from build123d import *

# Parameters (mm, degrees)
SKETCH2_W           = 121.6
SKETCH2_H           = 98.919653249
SKETCH2_R           = 2
BOSS_EXTRUDE1_DEPTH = 3
SKETCH3_W           = 3
SKETCH3_H           = 12.364956656
BOSS_EXTRUDE2_DEPTH = 3
CUT_EXTRUDE1_DEPTH  = 101.7


with BuildPart() as part:
    # Sketch2 → Boss-Extrude1 (new body)
    with BuildSketch(Plane(origin=(0, 0, 0), x_dir=(1, 0, 0), z_dir=(0, 1, 0))):
        with Locations((20.5, -5.540173376)):
            Rectangle(SKETCH2_W, SKETCH2_H)
        Polygon((41.25, 0), (0, 0), (0, 7.75), (-2, 7.75), (-3, 10.25), (-2, 12.75), (0, 12.75), (0, 20.5), (41.25, 20.5), align=None, mode=Mode.SUBTRACT)
        with Locations(Location((-4.7, 4.7, 0), (0, 0, 270))):
            Circle(SKETCH2_R, mode=Mode.SUBTRACT)
        with Locations(Location((-4.7, 15.8, 0), (0, 0, 270))):
            Circle(SKETCH2_R, mode=Mode.SUBTRACT)
        with Locations(Location((45.7, 4.7, 0), (0, 0, 270))):
            Circle(SKETCH2_R, mode=Mode.SUBTRACT)
        with Locations(Location((45.7, 15.8, 0), (0, 0, 270))):
            Circle(SKETCH2_R, mode=Mode.SUBTRACT)
    extrude(amount=BOSS_EXTRUDE1_DEPTH)

    # Sketch3 → Boss-Extrude2 (add, through all)
    with BuildSketch(Plane(origin=(0, 0, 0), x_dir=(1, 0, 0), z_dir=(0, 1, 0))):
        with Locations((-41.8, 26.736608875)):
            Rectangle(SKETCH3_W, SKETCH3_H)
        with Locations((-41.8, -6.236608875)):
            Rectangle(SKETCH3_W, SKETCH3_H)
        with Locations((82.8, -6.236608875)):
            Rectangle(SKETCH3_W, SKETCH3_H)
        with Locations((82.8, 26.736608875)):
            Rectangle(SKETCH3_W, SKETCH3_H)
    extrude(amount=BOSS_EXTRUDE2_DEPTH)

    # Sketch4 → Cut-Extrude1 (cut, through all)
    with BuildSketch(Plane(origin=(0, 0, 0), x_dir=(1, 0, 0), z_dir=(0, 1, 0))):
        Polygon((81.3, 8.75), (74.3, 8.75), (74.3, 7.25), (72.3, 7.25), (72.3, 13.25), (74.3, 13.25), (74.3, 11.75), (81.3, 11.75), align=None)
        Polygon((81.3, 30.348544885), (74.3, 30.348544885), (74.3, 28.848544885), (72.3, 28.848544885), (72.3, 34.848544885), (74.3, 34.848544885), (74.3, 33.348544885), (81.3, 33.348544885), align=None)
        Polygon((-40.3, 30.348544885), (-40.3, 33.348544885), (-33.3, 33.348544885), (-33.3, 34.848544885), (-31.3, 34.848544885), (-31.3, 28.848544885), (-33.3, 28.848544885), (-33.3, 30.348544885), align=None)
        Polygon((-40.3, 8.75), (-40.3, 11.75), (-33.3, 11.75), (-33.3, 13.25), (-31.3, 13.25), (-31.3, 7.25), (-33.3, 7.25), (-33.3, 8.75), align=None)
    extrude(amount=CUT_EXTRUDE1_DEPTH, mode=Mode.SUBTRACT)


solid = part.part
Build history of the part. All positions in model axes, mm. A direction names the side the tool comes from. Round coordinates to 2 decimals unless told otherwise and drop trailing zeros. Loops run counter-clockwise (first coordinate to the right, second up) from the corner with the lowest first, then second, coordinate; pieces in that order, holes last. Notation, with made-up numbers: (-8.5, 53) -> (42.5, 53) arc R15 ccw to (42.5, 65) -> close; hole circle Ø5 at (56.25, -22). An arc over 180 degrees is marked (long way). One line per item, written item: value. Start each with the question number.
Q1. Two-plate mould, pull along Z, no slides. Class faces 1 (the face through (83, 1, 12.419)), 2 (the face through (-43.3, 1, 6)), 3 (the face through (20, 1, -43.92)), 4 (the face through (-40.3, 1, -16)): released by +Z, released by -Z, zero draft, split by the parting line, or undercut.
Q2. Drop flat-ended pins along their axis: pin 1 Ø2 at (x, z) = (68, 21) entering from -Y; pin 2 Ø1.5 at (y, z) = (0.5, 23) entering from +X; pin 3 Ø0.9 at (y, z) = (1, -9) entering from -X. Give the stop position or say it passes through.
Q3. 3-axis set-ups, long thin cutter, end or side, ignore diameter. For faces 5 (the face through (-40.3, 1, 34)), 6 (the face through (-40.3, 1, -4)), 7 (the face through (-2.5, 1.5, -9)), 8 (the face through (83, 1, 0.054)): which of +Z, -Z, +X, -X, +Y, -Y reach the whole face in a straight line?
Q4. Cut at A-A on z = -4.7. List the corners of the cut face in (x, y).
Q5. Cut at B-B on x = 34. List the corners of the cut face in (y, z).
Q6. Probe line 1 along X through (y, z) = (1, -15.8); line 2 along Z through (x, y) = (-5, 0.45); line 3 along X through (y, z) = (0.7, -7.5). List the from-to ranges inside material, lowest first.
Q7. Cut at D-D on z = 46.5. List the corners of the cut face in (x, y).
Q8. Cut at C-C on y = 1.8. Count the separate pieces of the cut face and the enclosed holes in it, plus the area to 3 significant figures.
Computed:
1. face 1: released by +Z
1. face 2: zero draft
1. face 3: released by -Z
1. face 4: undercut
2. pin 1: y = 0
2. pin 2: x = 81.3
2. pin 3: x = -40.3
3. face 5: +Z, -X, +Y, -Y
3. face 6: -X, +Y, -Y
3. face 7: +Y, -Y
3. face 8: +X, +Y, -Y
4. outline: (-40.3, 0) -> (-6.7, 0) -> (-6.7, 3) -> (-40.3, 3) -> close; (-2.7, 0) -> (0, 0) -> (0, 3) -> (-2.7, 3) -> close; (41.25, 0) -> (43.7, 0) -> (43.7, 3) -> (41.25, 3) -> close; (47.7, 0) -> (81.3, 0) -> (81.3, 3) -> (47.7, 3) -> close
5. outline: (0, -43.92) -> (3, -43.92) -> (3, -20.5) -> (0, -20.5) -> close; (0, 0) -> (3, 0) -> (3, 55) -> (0, 55) -> close
6. line 1: -40.3 to -6.7, -2.7 to 0, 41.25 to 43.7, 47.7 to 81.3
6. line 2: -43.92 to -17.78, -13.82 to -6.68, -2.72 to 55
6. line 3: -40.3 to -33.3, -31.3 to 0, 41.25 to 72.3, 74.3 to 81.3
7. outline: (-40.3, 0) -> (81.3, 0) -> (81.3, 3) -> (-40.3, 3) -> close
8. separate pieces: 1
8. enclosed holes: 5
8. area: 11,100 mm²
